Verification items for the finished model (mm, model axes). Coordinates: 2 decimals unless noted, no trailing zeros. Order: outer loops, then holes, each group sorted by start corner. A loop starts at its lowest first (then second) coordinate and runs counter-clockwise, first axis right, second up. Notation, with made-up numbers: M -20,-7.75 L 16,-7.75 A31 cw 16,24.25 Z; hole C 46.25,11 d2. An arc over 180 degrees is marked long. Return JSON: item names as keys, results as strings. Group by question number.
Q1. Mould release check, pull along X, two halves, no side actions. Record for faces 1 (the face through (20.05, 3.04, 26.47)), 2 (the face through (-16.55, 3, 0)), 3 (the face through (-20.12, 3.04, 26.4)): pulls with the +X half, pulls with the -X half, needs draft (parallel to the pull), parting line crosses it, or undercut.
Q2. Section check B-B, the plane z = -8. Enter the section's corners in (x, y).
Q3. Section check A-A, the plane x = 15.5. Enter the section's corners in (y, z), then the cut area to 3 significant figures.
Q4. Section check D-D, the plane z = 0. Enter the section's corners in (x, y), then the cut area to 3 significant figures.
Q5. Thickness scan on probe 1 along Z at (x, y) = (0, 3.8); probe 2 along X at (y, z) = (3.7, 0); probe 3 along X at (y, z) = (3.5, -17.5) (3 decimals). Record the ranges inside material, lowest first.
Q6. Section check C-C, the plane x = 3.5. Enter the section's corners in (y, z).
from build123d import *

# Parameters (mm, degrees)
SKETCH1_W           = 43.1
SKETCH1_H           = 55.8
SKETCH1_R           = 1.75
SKETCH1_R_2         = 1.5
BOSS_EXTRUDE1_DEPTH = 6
FILLET3_R           = 5
FILLET4_R           = 1


with BuildPart() as part:
    # Sketch1 → Boss-Extrude1 (new body)
    with BuildSketch(Plane(origin=(0, 0, 0), x_dir=(1, 0, 0), z_dir=(0, 1, 0))):
        Rectangle(SKETCH1_W, SKETCH1_H)
        with Locations((11.375, 17.5)):
            Circle(SKETCH1_R, mode=Mode.SUBTRACT)
        with Locations((11.375, -17.5)):
            Circle(SKETCH1_R, mode=Mode.SUBTRACT)
        with Locations((-11.375, -17.5)):
            Circle(SKETCH1_R, mode=Mode.SUBTRACT)
        with Locations((-11.375, 17.5)):
            Circle(SKETCH1_R, mode=Mode.SUBTRACT)
        with Locations((0, 25.4)):
            Circle(SKETCH1_R_2, mode=Mode.SUBTRACT)
        with Locations((-19.05, 0)):
            Circle(SKETCH1_R_2, mode=Mode.SUBTRACT)
        with Locations((19.05, 0)):
            Circle(SKETCH1_R_2, mode=Mode.SUBTRACT)
        with Locations((0, -25.4)):
            Circle(SKETCH1_R_2, mode=Mode.SUBTRACT)
        Polygon((14.25, -14.25), (8.65, -14.25), (8.65, -20.75), (14.25, -20.75), (16.55, -20.75), (16.55, -22.9), (-16.55, -22.9), (-16.55, -20.75), (-14.25, -20.75), (-8.65, -20.75), (-8.65, -14.25), (-14.25, -14.25), (-16.55, -14.25), (-16.55, 14.25), (-14.25, 14.25), (-8.65, 14.25), (-8.65, 20.75), (-14.25, 20.75), (-16.55, 20.75), (-16.55, 22.9), (16.55, 22.9), (16.55, 20.75), (14.25, 20.75), (8.65, 20.75), (8.65, 14.25), (14.25, 14.25), (16.55, 14.25), (16.55, -14.25), align=None, mode=Mode.SUBTRACT)
    extrude(amount=BOSS_EXTRUDE1_DEPTH)

    # Fillet3
    fillet3_edges = [part.edges().sort_by_distance(p)[0] for p in [
        (-21.55, 3, 27.9),
        (-21.55, 3, -27.9),
        (21.55, 3, -27.9),
        (21.55, 3, 27.9),
    ]]
    fillet(fillet3_edges, radius=FILLET3_R)

    # Fillet4
    fillet4_edges = [part.edges().sort_by_distance(p)[0] for p in [
        (-8.65, 3, -20.75),
        (-8.65, 3, -14.25),
        (-8.65, 3, 14.25),
        (-8.65, 3, 20.75),
        (8.65, 3, 20.75),
        (8.65, 3, 14.25),
        (8.65, 3, -14.25),
        (8.65, 3, -20.75),
    ]]
    fillet(fillet4_edges, radius=FILLET4_R)


solid = part.part
Numbers:
{
 "1": {"face 1": "pulls with the +X half", "face 2": "undercut", "face 3": "pulls with the -X half"},
 "2": {"outline": "M -21.55,0 L -16.55,0 L -16.55,6 L -21.55,6 Z; M 16.55,0 L 21.55,0 L 21.55,6 L 16.55,6 Z"},
 "3": {"outline": "M 0,-27.9 L 6,-27.9 L 6,-22.9 L 0,-22.9 Z; M 0,-20.75 L 6,-20.75 L 6,-14.25 L 0,-14.25 Z; M 0,14.25 L 6,14.25 L 6,20.75 L 0,20.75 Z; M 0,22.9 L 6,22.9 L 6,27.9 L 0,27.9 Z", "area": "138 mm2"},
 "4": {"outline": "M -21.55,0 L -20.55,0 L -20.55,6 L -21.55,6 Z; M -17.55,0 L -16.55,0 L -16.55,6 L -17.55,6 Z; M 16.55,0 L 17.55,0 L 17.55,6 L 16.55,6 Z; M 20.55,0 L 21.55,0 L 21.55,6 L 20.55,6 Z", "area": "24.0 mm2"},
 "5": {"probe 1": "z = -27.9 to -26.9, -23.9 to -22.9, 22.9 to 23.9, 26.9 to 27.9", "probe 2": "x = -21.55 to -20.55, -17.55 to -16.55, 16.55 to 17.55, 20.55 to 21.55", "probe 3": "x = -21.55 to -13.125, -9.625 to -8.65, 8.65 to 9.625, 13.125 to 21.55"},
 "6": {"outline": "M 0,-27.9 L 6,-27.9 L 6,-22.9 L 0,-22.9 Z; M 0,22.9 L 6,22.9 L 6,27.9 L 0,27.9 Z"}
}
